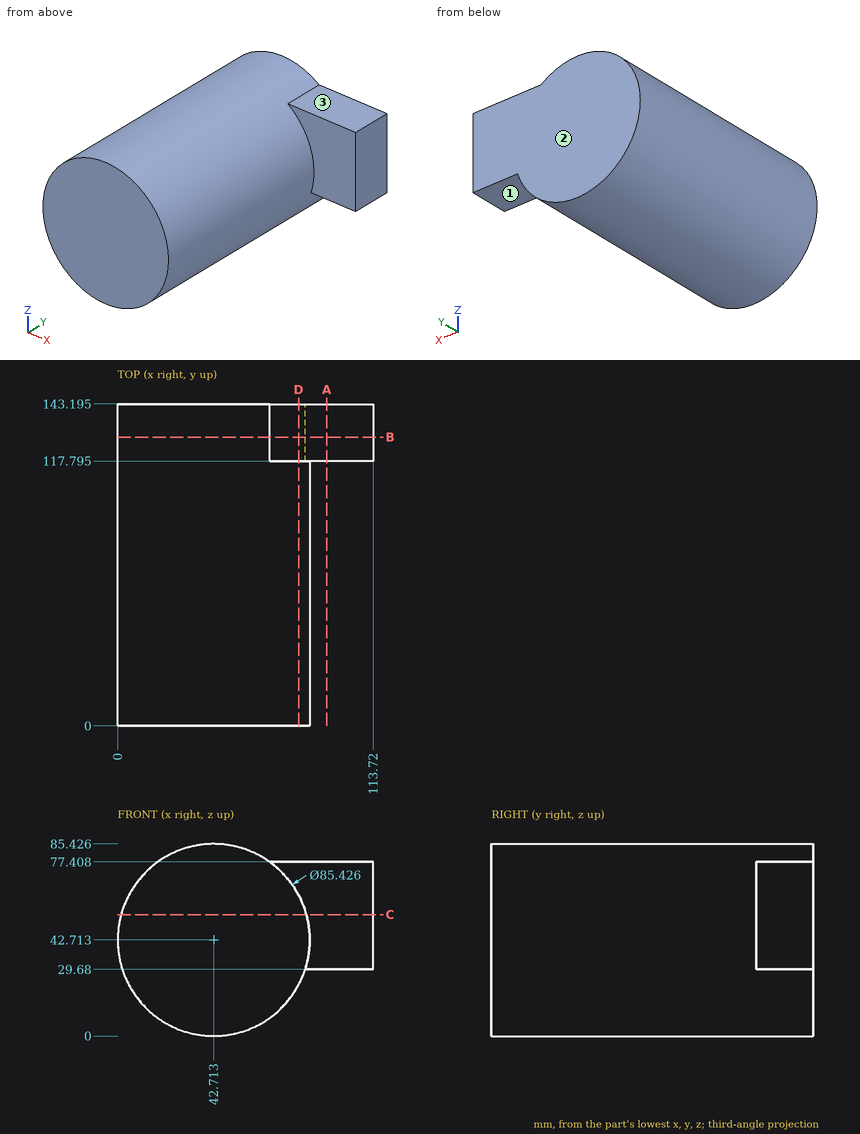
Geometry check sheet. Reference: drawing and pictorial views, mm from the part's lowest x, y, z. A direction names the side the tool comes from. Round coordinates to 2 decimals unless told otherwise and drop trailing zeros. Order: outer loops, then holes, each group sorted by start corner. A loop starts at its lowest first (then second) coordinate and runs counter-clockwise, first axis right, second up.
Q1. Depth check by flat-ended pin: P1, Ø12, axis at x = 92, z = 51, coming from the -Y side (1 decimal); P2, Ø10, axis at y = 94.5, z = 37, coming from the +X side; P3, Ø1, axis at y = 86.5, z = 30, coming from the -X side. Enter the tip coordinate at first touch or a pass-through.
Filled sheet:
P1: stops at y = 117.8
P2: stops at x = 85.42
P3: stops at x = 1.78
Q2. Cross-section at D-D, the plane x = 80.5. Enter the section's corners in (y, z) (1 decimal).
Filled sheet:
outline: (0, 22.8) - (143.2, 22.8) - (143.2, 77.4) - (117.8, 77.4) - (117.8, 62.6) - (0, 62.6) - close
Q3. Cross-section at C-C, the plane z = 54. Enter the section's corners in (x, y) (1 decimal), plus the area to 3 significant figures.
Filled sheet:
outline: (1.5, 0) - (83.9, 0) - (83.9, 117.8) - (113.7, 117.8) - (113.7, 143.2) - (1.5, 143.2) - close
area: 12,600 mm2
Q4. Cross-section at B-B, the plane y = 128.5. Enter the section's corners in (x, z), plus the area to 3 significant figures.
Filled sheet:
outline: (67.63, 77.41) arc R42.71 ccw (long way) to (83.39, 29.68) - (113.72, 29.68) - (113.72, 77.41) - close
area: 7,280 mm2
Q5. Scan lines: L1, parallel to Y at x = 92, z = 72 (1 decimal); L2, parallel to Z at x = 99.5, y = 125; L3, parallel to X at y = 98.5, z = 37.5. Record each from-to range of solid material in increasing order.
Filled sheet:
L1: y = 117.8 to 143.2
L2: z = 29.68 to 77.41
L3: x = 0.32 to 85.11
Q6. Cross-section at A-A, the plane x = 93. Enter the section's corners in (y, z) (1 decimal).
Filled sheet:
outline: (117.8, 29.7) - (143.2, 29.7) - (143.2, 77.4) - (117.8, 77.4) - close
Q7. Set-up check for the marked faces 1, 2 and 3: record each of +Z, -Z, +X, -X, +Y, -Y from which the full face is reachable in a straight line by a thin tool's end or side.
Filled sheet:
face 1: -Z, +X, +Y, -Y
face 2: +Z, -Z, +X, -X, +Y
face 3: +Z, +X, +Y, -Y
